from build123d import *

# Parameters (mm, degrees)
BOSS_EXTRUDE1_DEPTH = 10.1
BOSS_EXTRUDE2_DEPTH = 29.9
CUT_EXTRUDE1_DEPTH  = 6.1
CUT_EXTRUDE2_DEPTH  = 71.313654435


with BuildPart() as part:
    # Sketch1 → Boss-Extrude1 (new body)
    with BuildSketch(Plane(origin=(0, 0, 0), x_dir=(1, 0, 0), z_dir=(0, 1, 0))):
        Polygon((0, 0), (45, 0), (0, 45), align=None)
    extrude(amount=BOSS_EXTRUDE1_DEPTH)

    # Sketch2 → Boss-Extrude2 (add)
    with BuildSketch(Plane(origin=(0, 10.1, 0), x_dir=(1, 0, 0), z_dir=(0, 1, 0))):
        Polygon((0, 0), (45, 0), (41, 4), (4, 4), (4, 41), (0, 45), align=None)
    extrude(amount=BOSS_EXTRUDE2_DEPTH)

    # Sketch3 → Cut-Extrude1 (cut)
    with BuildSketch(Plane(origin=(0, 10.1, 0), x_dir=(1, 0, 0), z_dir=(0, 1, 0))):
        with BuildLine():
            Line((12.535533906, 28.221825407), (28.221825407, 12.535533906))
            ThreePointArc((28.221825407, 12.535533906), (28.221825407, 5.464466094), (21.150757595, 5.464466094))
            Line((21.150757595, 5.464466094), (5.464466094, 21.150757595))
            ThreePointArc((5.464466094, 21.150757595), (5.464466094, 28.221825407), (12.535533906, 28.221825407))
        make_face()
    extrude(amount=-CUT_EXTRUDE1_DEPTH, mode=Mode.SUBTRACT)

    # Sketch5 → Cut-Extrude2 (cut, through all)
    with BuildSketch(Plane(origin=(0, 10.1, 0), x_dir=(1, 0, 0), z_dir=(0, 1, 0))):
        with BuildLine():
            Line((10.944543648, 26.630835149), (26.630835149, 10.944543648))
            ThreePointArc((26.630835149, 10.944543648), (26.630835149, 7.055456352), (22.741747853, 7.055456352))
            Line((22.741747853, 7.055456352), (7.055456352, 22.741747853))
            ThreePointArc((7.055456352, 22.741747853), (7.055456352, 26.630835149), (10.944543648, 26.630835149))
        make_face()
    extrude(amount=-CUT_EXTRUDE2_DEPTH, mode=Mode.SUBTRACT)


solid = part.part
Input: part model. Units: mm. Frame: model coordinates. A direction names the side the tool comes from. Coordinates: 2 decimals unless noted, no trailing zeros. Loops run counter-clockwise (first coordinate to the right, second up) from the corner with the lowest first, then second, coordinate; pieces in that order, holes last.
(1) First-contact query: pin 1 Ø10 at (y, z) = (9.5, -14) entering from -X; pin 2 Ø12 at (x, z) = (29, -27) entering from +Y; pin 3 Ø6 at (x, z) = (9, -12) entering from +Y; pin 4 Ø6 at (y, z) = (32.5, -13.5) entering from +X. Flat tips, straight axial feed; report the tip coordinate or a pass-through.
(2) Material intervals for probe 1 along Y at (x, z) = (26, -16.5); probe 2 along X at (y, z) = (25, -29.5); probe 3 along Z at (x, y) = (6.5, 30), sorted ascending.
(3) Section C-C on y = 18. Return the cut outline in (x, z).
(4) Set-up query: faces 1 (the face through (13.417, 7.093, -13.198)), 2 (the face through (0, 20, -23)), 3 (the face through (4, 25, -22)), 4 (the face through (18.678, 2.028, -18.897)). Return all of +Z, -Z, +X, -X, +Y, -Y with unobstructed straight access to the full face (end or side cutting, diameter ignored); none if empty.
(5) Section B-B on x = 9. Return the cut outline in (y, z), then the cut area to 3 significant figures.
(6) Pull-direction query (Z, two-part tool) for faces 5 (the face through (22, 20, 0)), 6 (the face through (23, 6, -22)), 7 (the face through (7.013, 2.028, -26.588)), 8 (the face through (20, 10.1, -21)); classes: released by +Z, released by -Z, zero draft, split by the parting line, or undercut.
(7) Section A-A on z = -9. Return the cut outline in (x, y), then the cut area to 3 significant figures.
(8) Section D-D on z = -36. Return the cut outline in (x, y), then the cut area to 4 significant figures.
Data:
1. pin 1: stops at x = 0
1. pin 2: passes through
1. pin 3: stops at y = 10.1
1. pin 4: stops at x = 4
2. probe 1: y = 0 to 10.1
2. probe 2: x = 0 to 4
2. probe 3: z = -4 to 0
3. outline: (0, -45) - (4, -41) - (4, -4) - (41, -4) - (45, 0) - (0, 0) - close
4. face 1: +Y
4. face 2: +Z, -Z, -X, +Y, -Y
4. face 3: -Z, +X, +Y
4. face 4: +Y, -Y
5. outline: (0, -36) - (10.1, -36) - (10.1, -29.69) - (4, -29.69) - (4, -27.44) - (0, -27.44) - close; (0, -20.8) - (4, -20.8) - (4, -17.62) - (10.1, -17.62) - (10.1, -4) - (40, -4) - (40, 0) - (0, 0) - close
5. area: 383 mm2
6. face 5: released by +Z
6. face 6: released by -Z
6. face 7: undercut
6. face 8: zero draft
7. outline: (0, 0) - (20.8, 0) - (20.8, 4) - (17.62, 4) - (17.62, 10.1) - (4, 10.1) - (4, 40) - (0, 40) - close; (27.44, 0) - (36, 0) - (36, 10.1) - (29.69, 10.1) - (29.69, 4) - (27.44, 4) - close
7. area: 383 mm2
8. outline: (0, 0) - (9, 0) - (9, 10.1) - (4, 10.1) - (4, 40) - (0, 40) - close
8. area: 210.5 mm2
